```python
from build123d import *

# Parameters (mm, degrees)
BOSS_EXTRUDE1_START = 2.9
BOSS_EXTRUDE1_DEPTH = 7.167067
BOSS_EXTRUDE2_DEPTH = 1
CUT_EXTRUDE1_REACH  = 10.167
SKETCH3_R           = 0.9
CUT_EXTRUDE2_REACH  = 9.167
SKETCH4_R           = 1.6


with BuildPart() as part:
    # Sketch1 → Boss-Extrude1 (new body)
    with BuildSketch(Plane.XY.offset(BOSS_EXTRUDE1_START)):
        with BuildLine():
            Line((-4.955510048, -0.665522472), (-8.73567769, 27.481774602))
            ThreePointArc((-8.73567769, 27.481774602), (-4.445690114, 33.102807123), (1.175342406, 28.812819547))
            Line((1.175342406, 28.812819547), (4.955510048, 0.665522472))
            ThreePointArc((4.955510048, 0.665522472), (0.665522472, -4.955510048), (-4.955510048, -0.665522472))
        make_face()
    extrude(amount=BOSS_EXTRUDE1_DEPTH)

    # Sketch2 → Boss-Extrude2 (add)
    with BuildSketch(Plane(origin=(0, 0, 2.9), x_dir=(-1, 0, 0), z_dir=(0, 0, -1))):
        with BuildLine():
            Line((-3.624465104, 10.576542569), (-1.175342406, 28.812819547))
            ThreePointArc((-1.175342406, 28.812819547), (4.445690114, 33.102807123), (8.73567769, 27.481774602))
            Line((8.73567769, 27.481774602), (6.286554993, 9.245497624))
            Line((6.286554993, 9.245497624), (-3.624465104, 10.576542569))
        make_face()
    extrude(amount=BOSS_EXTRUDE2_DEPTH)

    # Sketch3 → Cut-Extrude1 (cut, up to next)
    with BuildSketch(Plane(origin=(0, 0, 1.9), x_dir=(-1, 0, 0), z_dir=(0, 0, -1)), mode=Mode.PRIVATE) as cut_extrude1_sk1:
        with Locations((3.780167642, 28.147297074)):
            Circle(SKETCH3_R)
    cut_extrude1_tool1 = extrude(cut_extrude1_sk1.sketch, amount=-CUT_EXTRUDE1_REACH, mode=Mode.PRIVATE) & part.part
    add(cut_extrude1_tool1.solids().sort_by_distance((-3.780168, 28.147297, 1.9))[0], mode=Mode.SUBTRACT)
    # Sketch3 → Cut-Extrude1 (cut, up to next)
    with BuildSketch(Plane(origin=(0, 0, 1.9), x_dir=(-1, 0, 0), z_dir=(0, 0, -1)), mode=Mode.PRIVATE) as cut_extrude1_sk2:
        with Locations((3.380854159, 25.173991045)):
            Circle(SKETCH3_R)
    cut_extrude1_tool2 = extrude(cut_extrude1_sk2.sketch, amount=-CUT_EXTRUDE1_REACH, mode=Mode.PRIVATE) & part.part
    add(cut_extrude1_tool2.solids().sort_by_distance((-3.380854, 25.173991, 1.9))[0], mode=Mode.SUBTRACT)
    # Sketch3 → Cut-Extrude1 (cut, up to next)
    with BuildSketch(Plane(origin=(0, 0, 1.9), x_dir=(-1, 0, 0), z_dir=(0, 0, -1)), mode=Mode.PRIVATE) as cut_extrude1_sk3:
        with Locations((2.981540675, 22.200685016)):
            Circle(SKETCH3_R)
    cut_extrude1_tool3 = extrude(cut_extrude1_sk3.sketch, amount=-CUT_EXTRUDE1_REACH, mode=Mode.PRIVATE) & part.part
    add(cut_extrude1_tool3.solids().sort_by_distance((-2.981541, 22.200685, 1.9))[0], mode=Mode.SUBTRACT)
    # Sketch3 → Cut-Extrude1 (cut, up to next)
    with BuildSketch(Plane(origin=(0, 0, 1.9), x_dir=(-1, 0, 0), z_dir=(0, 0, -1)), mode=Mode.PRIVATE) as cut_extrude1_sk4:
        with Locations((2.582227192, 19.227378987)):
            Circle(SKETCH3_R)
    cut_extrude1_tool4 = extrude(cut_extrude1_sk4.sketch, amount=-CUT_EXTRUDE1_REACH, mode=Mode.PRIVATE) & part.part
    add(cut_extrude1_tool4.solids().sort_by_distance((-2.582227, 19.227379, 1.9))[0], mode=Mode.SUBTRACT)
    # Sketch3 → Cut-Extrude1 (cut, up to next)
    with BuildSketch(Plane(origin=(0, 0, 1.9), x_dir=(-1, 0, 0), z_dir=(0, 0, -1)), mode=Mode.PRIVATE) as cut_extrude1_sk5:
        with Locations((2.182913709, 16.254072958)):
            Circle(SKETCH3_R)
    cut_extrude1_tool5 = extrude(cut_extrude1_sk5.sketch, amount=-CUT_EXTRUDE1_REACH, mode=Mode.PRIVATE) & part.part
    add(cut_extrude1_tool5.solids().sort_by_distance((-2.182914, 16.254073, 1.9))[0], mode=Mode.SUBTRACT)
    # Sketch3 → Cut-Extrude1 (cut, up to next)
    with BuildSketch(Plane(origin=(0, 0, 1.9), x_dir=(-1, 0, 0), z_dir=(0, 0, -1)), mode=Mode.PRIVATE) as cut_extrude1_sk6:
        with Locations((1.783600226, 13.280766929)):
            Circle(SKETCH3_R)
    cut_extrude1_tool6 = extrude(cut_extrude1_sk6.sketch, amount=-CUT_EXTRUDE1_REACH, mode=Mode.PRIVATE) & part.part
    add(cut_extrude1_tool6.solids().sort_by_distance((-1.7836, 13.280767, 1.9))[0], mode=Mode.SUBTRACT)

    # Sketch4 → Cut-Extrude2 (cut, up to next)
    with BuildSketch(Plane(origin=(0, 0, 2.9), x_dir=(-1, 0, 0), z_dir=(0, 0, -1)), mode=Mode.PRIVATE) as cut_extrude2_sk1:
        Circle(SKETCH4_R)
    cut_extrude2_tool1 = extrude(cut_extrude2_sk1.sketch, amount=-CUT_EXTRUDE2_REACH, mode=Mode.PRIVATE) & part.part
    add(cut_extrude2_tool1.solids().sort_by_distance((0, 0, 2.9))[0], mode=Mode.SUBTRACT)


solid = part.part
```
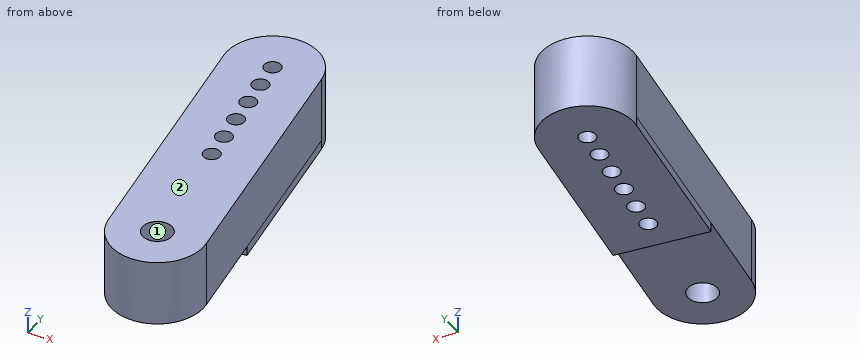
Check sheet for the modelled part. Datum: model origin and axes. Units: mm. Face numbers are marked on the shaded views. Give positions to 0.01 mm unless a question says otherwise; leave off trailing zeros. Loops run counter-clockwise (first coordinate to the right, second up) from the corner with the lowest first, then second, coordinate; pieces in that order, holes last. Notation, with made-up numbers: M 0.5,43.5 L 23.5,43.5 A21 ccw 23.5,54.5 Z; hole C 61,-10.5 d10. An arc over 180 degrees is marked long. Answer in a Markdown table with one row per item.
1) Cross-section at D-D (z = 6.25). Enter the section's corners in (x, y).
Solutions:
| item | result |
|---|---|
| outline | M -8.74,27.48 L -4.96,-0.67 A5 ccw 4.96,0.67 L 1.18,28.81 A5 ccw Z; hole C -3.78,28.15 d1.8; hole C -3.38,25.17 d1.8; hole C -2.98,22.2 d1.8; hole C -2.58,19.23 d1.8; hole C -2.18,16.25 d1.8; hole C -1.78,13.28 d1.8; hole C 0,0 d3.2 |
2) Cross-section at C-C (y = 0). Enter the section's corners in (x, z).
Solutions:
| item | result |
|---|---|
| outline | M -5.04,2.9 L -1.6,2.9 L -1.6,10.07 L -5.04,10.07 Z; M 1.6,2.9 L 5,2.9 L 5,10.07 L 1.6,10.07 Z |
3) Depth check by flat-ended pin: pin 1 (1.1 mm diameter, centred on x = -3.78, y = 28.15, fed in from +Z); pin 2 (2 mm diameter, centred on x = 3.5, y = 1, fed in from -Z); pin 3 (1.5 mm diameter, centred on y = 16, z = 4, fed in from +X); pin 4 (2 mm diameter, centred on y = 23, z = 8, fed in from +X). Enter the tip coordinate at first touch or a pass-through.
Solutions:
| item | result |
|---|---|
| pin 1 | passes through |
| pin 2 | stops at z = 2.9 |
| pin 3 | stops at x = 3 |
| pin 4 | stops at x = 2.09 |
4) Cross-section at A-A (x = 0). Enter the section's corners in (y, z), plus the area to 3 significant figures.
Solutions:
| item | result |
|---|---|
| outline | M -5,2.9 L -1.6,2.9 L -1.6,10.07 L -5,10.07 Z; M 1.6,2.9 L 10.09,2.9 L 10.09,1.9 L 31.42,1.9 L 31.42,10.07 L 1.6,10.07 Z |
| area | 259 mm^2 |
5) Cross-section at B-B (z = 2.5). Enter the section's corners in (x, y), plus the area to 3 significant figures.
Solutions:
| item | result |
|---|---|
| outline | M -8.74,27.48 L -6.29,9.25 L 3.62,10.58 L 1.18,28.81 A5 ccw Z; hole C -3.78,28.15 d1.8; hole C -3.38,25.17 d1.8; hole C -2.98,22.2 d1.8; hole C -2.58,19.23 d1.8; hole C -2.18,16.25 d1.8; hole C -1.78,13.28 d1.8 |
| area | 208 mm^2 |
6) Thickness scan on line 1 (Y direction, x = -1, z = 9.75); line 2 (Z direction, x = -0.5, y = 9); line 3 (Y direction, x = -2, z = 6.5). Record the ranges inside material, lowest first.
Solutions:
| item | result |
|---|---|
| line 1 | y = -4.9 to -1.25, 1.25 to 12.84, 13.72 to 32.3 |
| line 2 | z = 2.9 to 10.07 |
| line 3 | y = -4.58 to 12.41, 14.15 to 15.37, 17.14 to 18.54, 19.91 to 32.82 |
7) Mould release check, pull along Y, two halves, no side actions. Record for the marked faces 1 and 2: released by +Y, released by -Y, zero draft, split by the parting line, or undercut.
Solutions:
| item | result |
|---|---|
| face 1 | undercut |
| face 2 | zero draft |
